Read the model definition and answer for the solid it produces. Units are mm, in the model's axes. A direction names the side the tool comes from. Give positions to 0.01 mm unless a question says otherwise; leave off trailing zeros. Order: outer loops, then holes, each group sorted by start corner. A loop starts at its lowest first (then second) coordinate and runs counter-clockwise, first axis right, second up. Notation, with made-up numbers: (19.5, 25.25) - (52.5, 25.25) arc R17 ccw to (52.5, 46.25) - close; hole circle Ø2 at (13.25, -2.75). An arc over 180 degrees is marked (long way). Write item = value, one per line.
```python
from build123d import *

# Parameters (mm, degrees)
SKETCH_1_W                = 100
SKETCH_1_H                = 30
EXTRUDE_1_DEPTH           = 20
EXTRUDE_2_DEPTH           = 5
EXTRUDE_2_DEPTH_BACK      = 20
FILLET_1_R                = 5
CUT_EXTRUDE_1_DEPTH       = 8
SKETCH_4_R                = 1.5
CUT_EXTRUDE_2_DEPTH       = 95.599814737
HOLE_WIZARD_1_D           = 5
HOLE_WIZARD_1_CBORE_D     = 10
HOLE_WIZARD_1_CBORE_DEPTH = 6


with BuildPart() as part:
    # 草图1 → 凸台-拉伸1 (new body)
    with BuildSketch(Plane.XY):
        Rectangle(SKETCH_1_W, SKETCH_1_H)
    extrude(amount=EXTRUDE_1_DEPTH)

    # 草图2 → 凸台-拉伸2 (add, two sides: drawn at the far end of the back side and taken through both)
    with BuildSketch(Plane.XY.offset(20).offset(-EXTRUDE_2_DEPTH_BACK)):
        Polygon((50, -15), (70, -15), (90.695144291, 20.845041382), (50, 20.845041382), align=None)
    extrude(amount=EXTRUDE_2_DEPTH + EXTRUDE_2_DEPTH_BACK)

    # 圆角1
    fillet_1_edges = [part.edges().sort_by_distance(p)[0] for p in [
        (50, 15, 10),
        (50, 0, 20),
    ]]
    fillet(fillet_1_edges, radius=FILLET_1_R - 0.0001)  # a hair under: the kernel refuses the full size

    # 草图3 → 切除-拉伸1 (cut)
    with BuildSketch(Plane.XY.offset(25)):
        Polygon((75.695144291, 20.845041382), (68.195144291, 7.854660326), (83.195144291, 7.854660326), (90.695144291, 20.845041382), align=None)
    extrude(amount=-CUT_EXTRUDE_1_DEPTH, mode=Mode.SUBTRACT)

    # 草图4 → 切除-拉伸2 (cut, through all)
    with BuildSketch(Plane.XY.offset(17)):
        with Locations((80.319499944, 14.854660326)):
            Circle(SKETCH_4_R)
    extrude(amount=-CUT_EXTRUDE_2_DEPTH, mode=Mode.SUBTRACT)

    # 孔1 (through all)
    with Locations(Plane(origin=(61, 4.845041382, 25), x_dir=(1, 0, 0), z_dir=(0, 0, 1))):
        with Locations((0, 0)):
            CounterBoreHole(HOLE_WIZARD_1_D / 2, HOLE_WIZARD_1_CBORE_D / 2, HOLE_WIZARD_1_CBORE_DEPTH)


solid = part.part
```
1. Section D-D (x = -30) is taken. Determine the outline of the cut face in (y, z).
Recorded:
outline = (-15, 0) - (15, 0) - (15, 20) - (-15, 20) - close
2. Flat-ended cylindrical pins translate along their axes: pin 1 (1 mm diameter, centred on y = 0, z = 6.5, fed in from +X); pin 2 (8 mm diameter, centred on x = 61, y = 4.85, fed in from +Z); pin 3 (8 mm diameter, centred on y = 3.5, z = 6.5, fed in from +X). Find the tip coordinate at first contact, or state that the pin passes through.
Recorded:
pin_1 = 78.95
pin_2 = 19
pin_3 = 82.99
3. Section A-A (x = 61) is taken. Determine the outline of the cut face in (y, z), and give its area (3 significant figures).
Recorded:
outline = (-15, 0) - (2.35, 0) - (2.35, 19) - (-0.15, 19) - (-0.15, 25) - (-15, 25) - close; (7.35, 0) - (20.85, 0) - (20.85, 25) - (9.85, 25) - (9.85, 19) - (7.35, 19) - close
area = 741 mm^2
4. Determine the mould class of faces 4 (the face through (66, 3, 25)), 5 (the face through (-3, 15, 10)), 6 (the face through (63, 3, 19)), 7 (the face through (56.005, 5.065, 22.042)) for opening direction Y: +Y half, -Y half, draft (parallel to the pull), parting line (faces both ways), or undercut.
Recorded:
face_4 = draft
face_5 = +Y half
face_6 = undercut
face_7 = undercut
5. Section B-B (z = 4) is taken. Determine the outline of the cut face in (x, y).
Recorded:
outline = (-50, -15) - (70, -15) - (90.7, 20.85) - (50, 20.85) - (50, 20) arc R5 cw to (45, 15) - (-50, 15) - close; hole circle Ø5 at (61, 4.85); hole circle Ø3 at (80.32, 14.85)
6. For faces 1 (the face through (76, 7.855, 21)), 2 (the face through (-3, 0, 20)), 3 (the face through (50, 20.3, 12.4)), determine the directions among +Z, -Z, +X, -X, +Y, -Y from which every point of the face is accessible in a straight line to the end or side of a thin tool.
Recorded:
face_1 = +Z, +X
face_2 = +Z, -X, +Y, -Y
face_3 = +Z, -Z, -X, +Y
7. Straight lines are drawn through the part: L1, parallel to Y at x = 61, z = 21.2; L2, parallel to Z at x = 15, y = 7; L3, parallel to Y at x = 33, z = 9.5. For each, find the intervals that lie inside material, in ascending order. Write a range as [from, to].
Recorded:
L1 = [-15, -0.15], [9.85, 20.85]
L2 = [0, 20]
L3 = [-15, 15]
